from build123d import *

# Parameters (mm, degrees)
CUT_EXTRUDE1_DEPTH         = 11
FILLET1_R                  = 2
M2_5_TAPPED_HOLE1_D        = 2.05
M2_5_TAPPED_HOLE1_DEPTH    = 6.35
M2_5_TAPPED_HOLE1_TIP      = 0.615882135
SKETCH11_OUTSIDE_W         = 67.05
SKETCH11_OUTSIDE_H         = 67.05
CUT_EXTRUDE2_DEPTH         = 77.802868599
FILLET3_R                  = 2
CHAMFER1_SIZE              = 2
M4_TAPPED_HOLE1_AT_2_COUNT = 2
M4_TAPPED_HOLE1_AT_2_PITCH = 22
SKETCH15_R                 = 1.5
CUT_EXTRUDE4_DEPTH         = 10
SKETCH8_W                  = 1.65
SKETCH8_H                  = 40
M4_TAPPED_HOLE2_AT_2_COUNT = 2
M4_TAPPED_HOLE2_AT_2_PITCH = 32.908965344
M4_TAPPED_HOLE2_AT_3_COUNT = 2
M4_TAPPED_HOLE2_AT_3_PITCH = 32.908965344
CUT_EXTRUDE6_START         = 11
SKETCH17_R                 = 2.5
CUT_EXTRUDE6_DEPTH         = 4.001
SKETCH14_R                 = 2.15
CUT_EXTRUDE3_DEPTH         = 29.575


with BuildPart() as part:
    # Sketch1 → Revolve1 (revolve)
    with BuildSketch(Plane(origin=(0, 0, 0), x_dir=(0, 0, -1), z_dir=(1, 0, 0))):
        Polygon((13.2, 44.575), (13.2, 51.375), (15, 51.375), (15, 69.575), (23, 69.575), (23, 0), (13.2, 0), (9.5, 0), (9.5, 4), (15, 4), (15, 44.575), align=None)
    revolve(axis=Axis((0, 0, 0), (0, 1, 0)))

    # Sketch5 → Cut-Extrude1 (cut)
    with BuildSketch(Plane(origin=(0, 44.575, 0), x_dir=(-1, 0, 0), z_dir=(0, -1, 0))):
        with BuildLine():
            Line((-13.5, -18.62122445), (-13.5, -25.735977403))
            Line((-13.5, -25.735977403), (13.5, -25.735977403))
            Line((13.5, -25.735977403), (13.5, -18.62122445))
            ThreePointArc((13.5, -18.62122445), (16.584015432, -15.936449797), (19.14388926, -12.748))
            Line((19.14388926, -12.748), (13.93421226, -12.748))
            Line((13.93421226, -12.748), (11.092149393, -10.0977335))
            ThreePointArc((11.092149393, -10.0977335), (0, -15), (-11.092149393, -10.0977335))
            Line((-11.092149393, -10.0977335), (-13.93421226, -12.748))
            Line((-13.93421226, -12.748), (-19.14388926, -12.748))
            ThreePointArc((-19.14388926, -12.748), (-16.584015432, -15.936449797), (-13.5, -18.62122445))
        make_face()
        with BuildLine():
            Line((-7.5, -6.748), (-9.775605232, -8.870036209))
            ThreePointArc((-9.775605232, -8.870036209), (0, -13.2), (9.775605232, -8.870036209))
            Line((9.775605232, -8.870036209), (7.5, -6.748))
            Line((7.5, -6.748), (-7.5, -6.748))
        make_face()
    extrude(amount=CUT_EXTRUDE1_DEPTH, mode=Mode.SUBTRACT)

    # Fillet1
    fillet1_edges = [part.edges().sort_by_distance(p)[0] for p in [
        (11.092149393, 39.075, 10.0977335),
        (-11.092149393, 39.075, 10.0977335),
        (-13.93421226, 39.075, 12.748),
        (13.93421226, 39.075, 12.748),
    ]]
    fillet(fillet1_edges, radius=FILLET1_R)

    # M2.5 Tapped Hole1
    with Locations(Plane.XZ.offset(-44.575)):
        with Locations((-10.4775, 15.748), (10.4775, 15.748)):
            Hole(M2_5_TAPPED_HOLE1_D / 2, depth=M2_5_TAPPED_HOLE1_DEPTH)
            with Locations((0, 0, -(M2_5_TAPPED_HOLE1_DEPTH + M2_5_TAPPED_HOLE1_TIP / 2))):  # 118° drill point
                Cone(0, M2_5_TAPPED_HOLE1_D / 2, M2_5_TAPPED_HOLE1_TIP, mode=Mode.SUBTRACT)

    # Sketch11 outside → Cut-Extrude2 (cut, through all)
    with BuildSketch(Plane(origin=(0, 0, 0), x_dir=(1, 0, 0), z_dir=(0, 1, 0))):
        Rectangle(SKETCH11_OUTSIDE_W, SKETCH11_OUTSIDE_H)
        with BuildLine():
            Line((13.983717047, 18.260768263), (20.411593144, 10.600323832))
            ThreePointArc((20.411593144, 10.600323832), (0, -23), (-20.411593144, 10.600323832))
            Line((-20.411593144, 10.600323832), (-13.983717047, 18.260768263))
            ThreePointArc((-13.983717047, 18.260768263), (0, 23), (13.983717047, 18.260768263))
        make_face(mode=Mode.SUBTRACT)
    extrude(amount=CUT_EXTRUDE2_DEPTH, mode=Mode.SUBTRACT)

    # Fillet3
    fillet3_edges = [part.edges().sort_by_distance(p)[0] for p in [
        (13.983717047, 34.7875, -18.260768263),
        (-13.983717047, 34.7875, -18.260768263),
        (-20.411593144, 34.7875, -10.600323832),
        (20.411593144, 34.7875, -10.600323832),
    ]]
    fillet(fillet3_edges, radius=FILLET3_R)

    # Chamfer1
    chamfer1_edges = [part.edges().sort_by_distance(p)[0] for p in [
        (0, 69.575, 15),
    ]]
    chamfer(chamfer1_edges, length=CHAMFER1_SIZE)

    # Sketch12 → M4 Tapped Hole1 (revolve, cut)
    with BuildSketch(Plane(origin=(17.197655095, 42.575, -14.430546047), x_dir=(-0.6427876096865435, 0, -0.7660444431189747), z_dir=(0, 1, 0))):
        Polygon((0, 0), (0, 11.091420021), (1.65, 10.1), (1.65, 0), align=None)
    m4_tapped_hole1 = revolve(axis=Axis((22.062037309, 42.575, -18.512247369), (-0.7660444431189746, 0, 0.6427876096865436)), mode=Mode.SUBTRACT)

    # M4 Tapped Hole1 at 2: M4 Tapped Hole1 ×2
    with Locations(*[(0, i * M4_TAPPED_HOLE1_AT_2_PITCH, 0) for i in range(1, M4_TAPPED_HOLE1_AT_2_COUNT)]):
        add(m4_tapped_hole1, mode=Mode.SUBTRACT)

    # Mirror1: M4 Tapped Hole1 across plane
    add(m4_tapped_hole1.mirror(Plane(origin=(0, 0, 0), x_dir=(0, 0, 1), z_dir=(1, 0, 0))), mode=Mode.SUBTRACT)

    # Mirror1 copy 1 sketch → Mirror1 copy 1 (revolve, cut)
    with BuildSketch(Plane(origin=(-17.197655095, 64.575, -14.430546047), x_dir=(0.6427876096865435, 0, -0.7660444431189747), z_dir=(0, 1, 0))):
        Polygon((0, 0), (0, -11.091420021), (1.65, -10.1), (1.65, 0), align=None)
    revolve(axis=Axis((-22.062037309, 64.575, -18.512247369), (-0.7660444431189746, 0, -0.6427876096865436)), mode=Mode.SUBTRACT)

    # Sketch15 → Cut-Extrude4 (cut)
    with BuildSketch(Plane.XZ):
        with Locations(Location((-9.192388155, -9.192388155, 0), (0, 0, 270))):
            Circle(SKETCH15_R)
        with Locations(Location((-9.192388155, 9.192388155, 0), (0, 0, 270))):
            Circle(SKETCH15_R)
        with Locations(Location((9.192388155, 9.192388155, 0), (0, 0, 270))):
            Circle(SKETCH15_R)
        with Locations(Location((9.192388155, -9.192388155, 0), (0, 0, 270))):
            Circle(SKETCH15_R)
    extrude(amount=-CUT_EXTRUDE4_DEPTH, mode=Mode.SUBTRACT)


with BuildPart() as body_2:
    # Split1: the piece on the far side of the plane
    add(part.part)
    split(bisect_by=Plane.ZX.offset(29.575), keep=Keep.BOTTOM)

    # Sketch14 → Cut-Extrude3 (cut)
    with BuildSketch(Plane.XZ):
        with Locations(Location((-16.454482672, 9.5, 0), (0, 0, 270))):
            Circle(SKETCH14_R)
        with Locations(Location((16.454482672, 9.5, 0), (0, 0, 270))):
            Circle(SKETCH14_R)
        with Locations(Location((0, -19, 0), (0, 0, 270))):
            Circle(SKETCH14_R)
    extrude(amount=-CUT_EXTRUDE3_DEPTH, mode=Mode.SUBTRACT)


with BuildPart() as part_1:
    add(part.part)

    # Split1
    split(bisect_by=Plane.ZX.offset(29.575), keep=Keep.TOP)

    # Sketch8 → M4 Tapped Hole2 (revolve, cut)
    with BuildSketch(Plane(origin=(-16.454482672, 69.575, 9.5), x_dir=(0, 0, 1), z_dir=(1, 0, 0))):
        with Locations((0.825, 20)):
            Rectangle(SKETCH8_W, SKETCH8_H)
    m4_tapped_hole2 = revolve(axis=Axis((-16.454482672, 75.925, 9.5), (0, -1, 0)), mode=Mode.SUBTRACT)

    # M4 Tapped Hole2 at 2: M4 Tapped Hole2 ×2
    with Locations(*[Vector(0.499999999999998, 0, -0.8660254037844398) * (i * M4_TAPPED_HOLE2_AT_2_PITCH) for i in range(1, M4_TAPPED_HOLE2_AT_2_COUNT)]):
        add(m4_tapped_hole2, mode=Mode.SUBTRACT)

    # M4 Tapped Hole2 at 3: M4 Tapped Hole2 ×2
    with Locations(*[(i * M4_TAPPED_HOLE2_AT_3_PITCH, 0, 0) for i in range(1, M4_TAPPED_HOLE2_AT_3_COUNT)]):
        add(m4_tapped_hole2, mode=Mode.SUBTRACT)

    # Sketch17 → Cut-Extrude6 (cut)
    with BuildSketch(Plane.XZ.offset(-44.575).offset(CUT_EXTRUDE6_START)):
        with Locations(Location((10.4775, 15.748, 0), (0, 0, 90))):
            Circle(SKETCH17_R)
        with Locations(Location((-10.4775, 15.748, 0), (0, 0, 90))):
            Circle(SKETCH17_R)
    extrude(amount=CUT_EXTRUDE6_DEPTH, mode=Mode.SUBTRACT)


solid = part_1.part
Geometry check sheet. Reference: the model listing, model coordinates, mm. A direction names the side the tool comes from. Round coordinates to 2 decimals unless told otherwise and drop trailing zeros. Order: outer loops, then holes, each group sorted by start corner. A loop starts at its lowest first (then second) coordinate and runs counter-clockwise, first axis right, second up. Notation, with made-up numbers: M 22,44 L 80,44 A12 cw 80,67 Z; hole C 4,-35 d7. An arc over 180 degrees is marked long. Answer in a Markdown table with one row per item. Add a question column.
Item 1: Sectioned sample at B-B, the plane z = 0. Enter the section's corners in (x, y) (3 decimals).
Item 2: Material ranges on L1, parallel to Z at x = 0, y = 59.5; L2, parallel to X at y = 60, z = 9.5; L3, parallel to X at y = 56, z = 0, recorded low to high. Write a range as [from, to].
Item 3: Sectioned sample at A-A, the plane x = 0. Enter the section's corners in (y, z) (3 decimals).
Item 4: Depth check by flat-ended pin: pin 1 Ø10 at (x, z) = (-12, 7) entering from +Y (3 decimals); pin 2 Ø18 at (x, z) = (0, 0) entering from +Y; pin 3 Ø6 at (x, y) = (-0.5, 36) entering from -Z; pin 4 Ø2 at (x, y) = (17, 53) entering from -Z. Enter the tip coordinate at first touch or a pass-through.
Item 5: Set-up check for faces 1 (the face through (17, 39, 12.748)), 2 (the face through (-4.506, 37.18, -14.307)), 3 (the face through (0, 44.575, 14)): record each of +Z, -Z, +X, -X, +Y, -Y from which the full face is reachable in a straight line by a thin tool's end or side.
Item 6: Sectioned sample at D-D, the plane y = 37. Enter the section's corners in (x, z), plus the area to 3 significant figures.
Item 7: Sectioned sample at C-C, the plane y = 59. Enter the section's corners in (x, z).
Item 8: Draft check along Z on faces 4 (the face through (0, 49, -23)), 5 (the face through (15.063, 49.295, 10.387)), 6 (the face through (10, 51.375, 9)), 7 (the face through (13.979, 38.998, 12.605)). Enter one of: released by +Z, released by -Z, zero draft, split by the parting line, or undercut.
Filled in:
| question | item | result |
|---|---|---|
| 1 | outline | M -23,29.575 L -15,29.575 L -15,44.575 L -13.2,44.575 L -13.2,51.375 L -15,51.375 L -15,67.575 L -17,69.575 L -23,69.575 Z; M 13.2,44.575 L 15,44.575 L 15,29.575 L 23,29.575 L 23,69.575 L 17,69.575 L 15,67.575 L 15,51.375 L 13.2,51.375 Z |
| 2 | L1 | z = [-23, -20.65], [-17.35, -15], [15, 23] |
| 2 | L2 | x = [-20.95, -18.1], [-14.8, -11.61], [11.61, 14.8], [18.1, 20.95] |
| 2 | L3 | x = [-23, -15], [15, 23] |
| 3 | outline | M 29.575,-23 L 69.575,-23 L 69.575,-20.65 L 29.575,-20.65 Z; M 29.575,-17.35 L 69.575,-17.35 L 69.575,-17 L 67.575,-15 L 51.375,-15 L 51.375,-13.2 L 44.575,-13.2 L 44.575,-15 L 29.575,-15 Z; M 29.575,15 L 33.575,15 L 33.575,23 L 29.575,23 Z; M 44.575,13.2 L 51.375,13.2 L 51.375,15 L 67.575,15 L 69.575,17 L 69.575,23 L 44.575,23 Z |
| 4 | pin 1 | stops at y = 69.575 |
| 4 | pin 2 | passes through |
| 4 | pin 3 | stops at z = -23 |
| 4 | pin 4 | stops at z = -15.86 |
| 5 | face 1 | +Z, +X, -X |
| 5 | face 2 | -Y |
| 5 | face 3 | none |
| 6 | outline | M -20.52,-10.39 A2 ccw -20.27,-10.77 L -14.13,-18.09 A2 ccw -13.8,-18.4 A23 ccw 13.8,-18.4 A2 ccw 14.13,-18.09 L 20.27,-10.77 A2 ccw 20.52,-10.39 A23 ccw 19.14,12.75 L 14.72,12.75 A2 ccw 13.36,12.21 L 12.45,11.37 A2 ccw 12.19,8.74 A15 cw long -12.19,8.74 A2 ccw -12.45,11.37 L -13.36,12.21 A2 ccw -14.72,12.75 L -19.14,12.75 A23 ccw Z; hole C -16.45,9.5 d3.3; hole C 0,-19 d3.3; hole C 16.45,9.5 d3.3 |
| 6 | area | 653 mm² |
| 7 | outline | M -20.52,-10.39 A2 ccw -20.27,-10.77 L -14.13,-18.09 A2 ccw -13.8,-18.4 A23 ccw 13.8,-18.4 A2 ccw 14.13,-18.09 L 20.27,-10.77 A2 ccw 20.52,-10.39 A23 ccw long Z; hole C -16.45,9.5 d3.3; hole C 0,0 d30; hole C 0,-19 d3.3; hole C 16.45,9.5 d3.3 |
| 8 | face 4 | released by -Z |
| 8 | face 5 | undercut |
| 8 | face 6 | undercut |
| 8 | face 7 | released by +Z |
